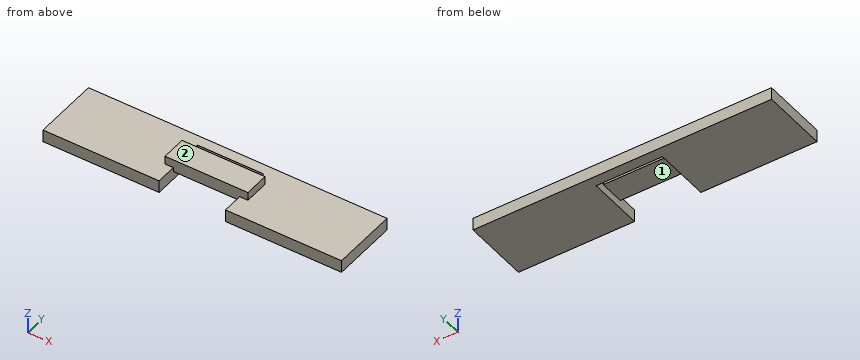
```python
from build123d import *

# Parameters (mm, degrees)
F0_W      = 57.15
F0_H      = 12.7
F1_DEPTH  = 2.38125
F2_W      = 15.875
F2_H      = 4.7625
F3_DEPTH  = 1.5875
F5_W      = 12.7
F5_H      = 4.7625
F6_DEPTH  = 3.175
F7_W      = 12.7
F7_H      = 3.96875
F8_DEPTH  = 2.38225
F9_W      = 12.7
F9_H      = 2
F10_DEPTH = 2.38225
F11_W     = 12.7
F11_H     = 4.7625
F12_DEPTH = 1.5875


# Not quite as in the source:
# - a feature of the source that left no trace in its solid (it failed there, or was rolled back) is left out
# - a length typed as a fraction of an inch, garbled in the dataset ("3 / 203.2 mm" for 3/8 in), is restored


with BuildPart() as f1:
    # F0 (on Top) → F1 (new body)
    with BuildSketch(Plane.XY):
        Rectangle(F0_W, F0_H)
    extrude(amount=F1_DEPTH)

    # F2 (on face) → F3 (join)
    with BuildSketch(Plane.XY.offset(2.38125)):
        Rectangle(F2_W, F2_H)
    extrude(amount=F3_DEPTH)

    # F5 (on offset) → F6 (cut, through all)
    with BuildSketch(Plane.XY.offset(3.175)):
        Rectangle(F5_W, F5_H)
    extrude(amount=-F6_DEPTH, mode=Mode.SUBTRACT)

    # F7 (on face) → F8 (cut, through all)
    with BuildSketch(Plane.XY.offset(2.38125)):
        with Locations((0, -4.365625)):
            Rectangle(F7_W, F7_H)
    extrude(amount=-F8_DEPTH, mode=Mode.SUBTRACT)

    # F9 (on face) → F10 (cut, through all)
    with BuildSketch(Plane.XY.offset(2.38125)):
        with Locations((0, 3.38125)):
            Rectangle(F9_W, F9_H)
    extrude(amount=-F10_DEPTH, mode=Mode.SUBTRACT)

    # F11 (on face) → F12 (join)
    with BuildSketch(Plane(origin=(0, 0, 3.175), x_dir=(1, 0, 0), z_dir=(0, 0, -1))):
        Rectangle(F11_W, F11_H)
    extrude(amount=F12_DEPTH)


solid = f1.part
```
Check sheet for the modelled part. Datum: model origin and axes. Units: mm. Face numbers are marked on the shaded views. A direction names the side the tool comes from. Coordinates: 2 decimals unless noted, no trailing zeros. Order: outer loops, then holes, each group sorted by start corner. A loop starts at its lowest first (then second) coordinate and runs counter-clockwise, first axis right, second up. Notation, with made-up numbers: M 23.25,58.5 L 52.25,58.5 A17 ccw 52.25,87.5 Z; hole C 51,30 d6. An arc over 180 degrees is marked long. Write each question's results on one line, items separated by ' | '. Start each with the question number.
1. Cross-section at B-B on y = -4. Record the cut outline in (x, z) (3 decimals), and give its area (3 significant figures).
2. Access from +Z, -Z, +X, -X, +Y, -Y to the whole of each face (thin tool, end or side, straight path). Record for the marked faces 1 and 2.
3. Cross-section at A-A on x = -1. Record the cut outline in (y, z), and give its area (3 significant figures).
4. Go/stop test with flat-tipped pins: P1, Ø1, axis at y = 1, z = 3, coming from the -X side; P2, Ø1.9, axis at x = 2, z = 0.5, coming from the -Y side; P3, Ø2.5, axis at x = -3, y = 1, coming from the -Z side. Record where each tip stops, or that it passes through.
5. Cross-section at D-D on x = 12. Record the cut outline in (y, z).
6. Material ranges on probe 1 along X at (y, z) = (2, 1.55) (3 decimals); probe 2 along Z at (x, y) = (-17, 0); probe 3 along Y at (x, z) = (0.5, 1.8), recorded low to high.
Checks:
1) outline: M -28.575,0 L -6.35,0 L -6.35,2.381 L -28.575,2.381 Z; M 6.35,0 L 28.575,0 L 28.575,2.381 L 6.35,2.381 Z | area: 106 mm²
2) face 1: -Z, -Y | face 2: +Z, +X, -X, +Y, -Y
3) outline: M -2.38,1.59 L 2.38,1.59 L 2.38,3.97 L -2.38,3.97 Z; M 4.38,0 L 6.35,0 L 6.35,2.38 L 4.38,2.38 Z | area: 16.0 mm²
4) P1: stops at x = -7.94 | P2: stops at y = 4.38 | P3: stops at z = 1.59
5) outline: M -6.35,0 L 6.35,0 L 6.35,2.38 L -6.35,2.38 Z
6) probe 1: x = -28.575 to -6.35, 6.35 to 28.575 | probe 2: z = 0 to 2.38 | probe 3: y = -2.38 to 2.38, 4.38 to 6.35
